Drawing for the job (mm, zero at the part's lowest x, y, z). A direction names the side the tool comes from. Round coordinates to 2 decimals unless told otherwise and drop trailing zeros. Loops run counter-clockwise (first coordinate to the right, second up) from the corner with the lowest first, then second, coordinate; pieces in that order, holes last.
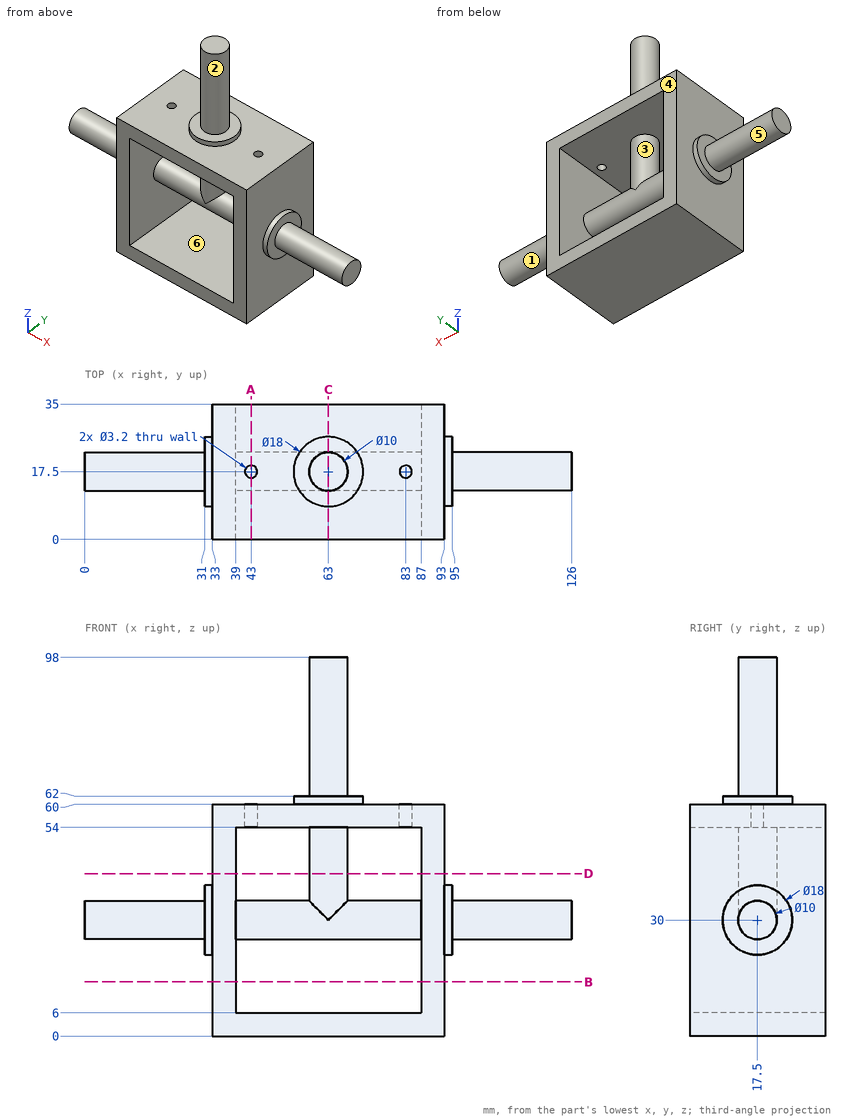
Q1. Slice it at D-D on z = 42. Give the cut face in (x, y), plus the area to 3 significant figures.
Q2. Probe line 1 (Y direction, x = 43, z = 56); line 2 (X direction, y = 13, z = 52); line 3 (X direction, y = 30.5, z = 7). List the from-to ranges inside material, lowest first.
Q3. Slice it at C-C on x = 63. Give the cut face in (y, z), plus the area to 3 significant figures.
Q4. Flat gauge pins, fed straight in: P1, Ø5, axis at x = 85, y = 8, coming from the +Z side; P2, Ø1.5, axis at y = 21.5, z = 52.5, coming from the +X side; P3, Ø10.5, axis at y = 20.5, z = 16, coming from the -X side. Where does each tip first touch, or does it go through?
Q5. Tool access for the marked faces 1, 2 and 3: list every direction of +Z, -Z, +X, -X, +Y, -Y with a clear straight run to the whole face (end or side of a thin tool).
Q6. Slice it at B-B on z = 14. Give the cut face in (x, y), plus the area to 3 significant figures.
Q7. Pull direction Z, two halves, no side cores. Call the marked faces 4, 5 and 6: pulls with the +Z half, pulls with the -Z half, needs draft (parallel to the pull), parting line crosses it, or undercut.
Q8. Slice it at A-A on x = 43. Give the cut face in (y, z).
Reply:
1. outline: (33, 0) - (39, 0) - (39, 35) - (33, 35) - close; circle Ø10 at (63, 17.5); (87, 0) - (93, 0) - (93, 35) - (87, 35) - close
1. area: 499 mm2
2. line 1: y = 0 to 15.9, 19.1 to 35
2. line 2: x = 33 to 39, 60.82 to 65.18, 87 to 93
2. line 3: x = 33 to 39, 87 to 93
3. outline: (0, 0) - (35, 0) - (35, 6) - (0, 6) - close; (0, 54) - (12.5, 54) - (12.5, 30) arc R5 ccw to (22.5, 30) - (22.5, 54) - (35, 54) - (35, 60) - (26.5, 60) - (26.5, 62) - (22.5, 62) - (22.5, 98) - (12.5, 98) - (12.5, 62) - (8.5, 62) - (8.5, 60) - (0, 60) - close
3. area: 1,100 mm2
4. P1: stops at z = 60
4. P2: stops at x = 93
4. P3: stops at x = 33
5. face 1: +X
5. face 2: +Z
5. face 3: none
6. outline: (33, 0) - (39, 0) - (39, 35) - (33, 35) - close; (87, 0) - (93, 0) - (93, 35) - (87, 35) - close
6. area: 420 mm2
7. face 4: needs draft
7. face 5: parting line crosses it
7. face 6: undercut
8. outline: (0, 0) - (35, 0) - (35, 6) - (0, 6) - close; (0, 54) - (15.9, 54) - (15.9, 60) - (0, 60) - close; circle Ø10 at (17.5, 30); (19.1, 54) - (35, 54) - (35, 60) - (19.1, 60) - close
